```python
from build123d import *

# Parameters (mm, degrees)
F0_R     = 6.5
F0_R_2   = 3
F1_DEPTH = 1
F2_DEPTH = 3
F3_R     = 0.99999
F4_R     = 0.5


# Not quite as in the source:
# - a fillet or chamfer is up to 0.001 mm smaller than in the source, because OpenCascade refuses the exact size


with BuildPart() as f1:
    # F0 (on Top) → F1 (new body)
    with BuildSketch(Plane.XY):
        Circle(F0_R)
        Circle(F0_R_2, mode=Mode.SUBTRACT)
    extrude(amount=F1_DEPTH)

    # F0 (on Top) → F2 (join)
    with BuildSketch(Plane.XY):
        Circle(F0_R_2)
    extrude(amount=F2_DEPTH)

    # F3 (radius 1 in the source; OpenCascade refuses exactly that, so slightly less here)
    f3_edges = [f1.edges().sort_by_distance(p)[0] for p in [
        (-6.5, 0, 0),
    ]]
    fillet(f3_edges, radius=F3_R)

    # F4
    f4_edges = [f1.edges().sort_by_distance(p)[0] for p in [
        (-3, 0, 3),
    ]]
    fillet(f4_edges, radius=F4_R)


solid = f1.part
```
Geometry: final body of the model. Coordinates: model frame, mm. Round coordinates to 2 decimals unless told otherwise and drop trailing zeros. Write each loop counter-clockwise with the first axis right and the second up, starting at its lowest first coordinate (ties: lowest second). Pieces come first, ordered by that corner, then holes.
Item 1: Material intervals for L1, parallel to Z at x = 1.5, y = 3.75; L2, parallel to Y at x = 2, z = 2.5; L3, parallel to X at y = -2.25, z = 0.9, sorted ascending.
Item 2: Section query C-C (z = 1.5). Return loops of the section in (x, y).
Item 3: Pin query (flat end, axial travel): P1, Ø1, axis at y = 4, z = 1, coming from the +X side. Return the tip coordinate at first contact, or that it passes through.
Item 4: Mould query, pull axis Y, two halves, no side actions, for faces 1 (the face through (3, -1, 1)), 2 (the face through (-3, 0, 2)). Classes: +Y half, -Y half, draft (parallel to the pull), parting line (faces both ways), or undercut.
Completed:
1. L1: z = 0 to 1
1. L2: y = -2.24 to 2.24
1. L3: x = -6.09 to 6.09
2. outline: circle Ø6 at (0, 0)
3. P1: stops at x = 5.48
4. face 1: draft
4. face 2: parting line
